The listing builds one solid part. Answer for the finished solid, in the listing's coordinates (mm). Give positions to 0.01 mm unless a question says otherwise; leave off trailing zeros. Write each loop counter-clockwise with the first axis right and the second up, starting at its lowest first coordinate (ties: lowest second). Pieces come first, ordered by that corner, then holes. Notation, with made-up numbers: (-2.75, -21.75) - (25.25, -21.75) arc R22 ccw to (25.25, 5.25) - close; hole circle Ø8 at (83, 82). An arc over 180 degrees is marked (long way). Return JSON: item names as keys, results as strings.
Autodesk Inventor part; units mm, degrees
ref_plane "YZ Plane" through (0, 0, 0) normal (1, 0, 0) x (0, 1, 0)
ref_plane "XZ Plane" through (0, 0, 0) normal (0, 1, 0) x (-1, 0, 0)
ref_plane "XY Plane" through (0, 0, 0) normal (0, 0, 1) x (1, 0, 0)
sketch "Boceto1" plane through (0, 0, 0) normal (0, 0, 1) x (1, 0, 0)
  line L0 (5, 0) -> (30, 0)
  line L1 (35, 5) -> (35, 60)
  line L2 (30, 65) -> (5, 65)
  line L3 (0, 60) -> (0, 5)
  arc A0 (5, 65) -> (0, 60) centre (5, 60) ccw
  arc A1 (35, 60) -> (30, 65) centre (30, 60) ccw
  arc A2 (0, 5) -> (5, 0) centre (5, 5) ccw
  arc A3 (30, 0) -> (35, 5) centre (30, 5) ccw
  circle A4 centre (17.5, 55) radius 4.5
  circle A5 centre (29, 48.25) radius 1.25
  circle A6 centre (29, 61.75) radius 1.25
  circle A7 centre (6, 61.75) radius 1.25
  circle A8 centre (6, 48.25) radius 1.25
  circle A9 centre (5, 8.75) radius 2.5
  circle A10 centre (30, 8.75) radius 2.5
  point P0 (0, 0)
extrude "Extrusión1" add sketch "Boceto1" along normal blind 3
sketch "Boceto2" plane through (0, 0, 3) normal (0, 0, 1) x (1, 0, 0)
  circle A0 centre (17.5, 55) radius 4.5
  circle A1 centre (29, 48.25) radius 1.25
  line L0 (29, 48.25) -> (29, 55)
  circle A2 centre (29, 61.75) radius 1.25
  line L1 (29, 55) -> (29, 61.75)
  circle A3 centre (6, 61.75) radius 1.25
  line L2 (29, 61.75) -> (6, 61.75)
  line L3 (17.5, 55) -> (29, 55)
  point P0 (0, 0)
  dimension "d20" = 23
  dimension "d21" = 6.75
  dimension "d22" = 11.5
properties part number "5"
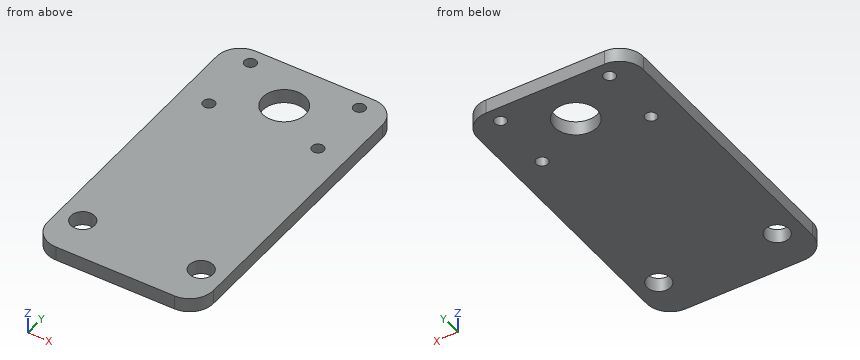
Item 1: Consider L1, parallel to Y at x = 17.5, z = 1; L2, parallel to Y at x = 30, z = 2.35; L3, parallel to X at y = 48, z = 0.6. Determine where each line is inside the solid, lowest interval first.
Answer below:
{"L1": "y = 0 to 50.5, 59.5 to 65", "L2": "y = 0 to 6.25, 11.25 to 47.5, 49 to 61, 62.5 to 65", "L3": "x = 0 to 4.78, 7.22 to 27.78, 30.22 to 35"}
Item 2: A cutting plane is placed at C-C on y = 55. Determine the outline of the cut face in (x, z), then the cut area to 3 significant figures.
Answer below:
{"outline": "(0, 0) - (13, 0) - (13, 3) - (0, 3) - close; (22, 0) - (35, 0) - (35, 3) - (22, 3) - close", "area": "78.0 mm²"}
Item 3: A cutting plane is placed at D-D on z = 2.35. Determine the outline of the cut face in (x, y), then the cut area to 3 significant figures.
Answer below:
{"outline": "(0, 5) arc R5 ccw to (5, 0) - (30, 0) arc R5 ccw to (35, 5) - (35, 60) arc R5 ccw to (30, 65) - (5, 65) arc R5 ccw to (0, 60) - close; hole circle Ø5 at (5, 8.75); hole circle Ø2.5 at (6, 48.25); hole circle Ø2.5 at (6, 61.75); hole circle Ø9 at (17.5, 55); hole circle Ø5 at (30, 8.75); hole circle Ø2.5 at (29, 48.25); hole circle Ø2.5 at (29, 61.75)", "area": "2,130 mm²"}
Item 4: Flat-ended cylindrical pins translate along their axes: P1, Ø4, axis at x = 29, y = 48.25, coming from the +Z side; P2, Ø1.5, axis at x = 4, z = 1, coming from the +Y side. Find the tip coordinate at first contact, or state that the pin passes through.
Answer below:
{"P1": "stops at z = 3", "P2": "stops at y = 64.99"}
Item 5: A cutting plane is placed at A-A on y = 8.75. Determine the outline of the cut face in (x, z), then the cut area to 3 significant figures.
Answer below:
{"outline": "(0, 0) - (2.5, 0) - (2.5, 3) - (0, 3) - close; (7.5, 0) - (27.5, 0) - (27.5, 3) - (7.5, 3) - close; (32.5, 0) - (35, 0) - (35, 3) - (32.5, 3) - close", "area": "75.0 mm²"}
Item 6: A cutting plane is placed at B-B on x = 15. Determine the outline of the cut face in (y, z).
Answer below:
{"outline": "(0, 0) - (51.26, 0) - (51.26, 3) - (0, 3) - close; (58.74, 0) - (65, 0) - (65, 3) - (58.74, 3) - close"}
